Autodesk Inventor part; units mm, degrees
ref_plane "YZ Plane" through (0, 0, 0) normal (1, 0, 0) x (0, 1, 0)
ref_plane "XZ Plane" through (0, 0, 0) normal (0, 1, 0) x (-1, 0, 0)
ref_plane "XY Plane" through (0, 0, 0) normal (0, 0, 1) x (1, 0, 0)
sketch "Skizze1" plane through (0, 0, 0) normal (0, 0, 1) x (1, 0, 0)
  line L0 (-914, 455) -> (914, 455)
  line L1 (914, 455) -> (914, -455)
  line L2 (914, -455) -> (-914, -455)
  line L3 (-914, -455) -> (-914, 455)
  line L4 (-914, 455) -> (914, -455) construction
  line L5 (914, 455) -> (-914, -455) construction
  line L6 (-901.5, -442.5) -> (901.5, -442.5)
  line L7 (901.5, -442.5) -> (901.5, 442.5)
  line L8 (901.5, 442.5) -> (-901.5, 442.5)
  line L9 (-901.5, 442.5) -> (-901.5, -442.5)
  line L10 (-901.5, -442.5) -> (901.5, 442.5) construction
  line L11 (901.5, -442.5) -> (-901.5, 442.5) construction
  point P0 (0, 0)
  dimension "d0" = 1828
  dimension "d1" = 910
  dimension "d2" = 1803
  dimension "d3" = 885
extrude "Extrusion1" add sketch "Skizze1" along normal blind 139
sketch "Skizze2" plane through (0, 0, 139) normal (0, 0, 1) x (1, 0, 0)
  line L0 (-901.5, 442.5) -> (901.5, 442.5)
  line L1 (-901.5, -442.5) -> (-901.5, 442.5)
  line L2 (901.5, -442.5) -> (-901.5, -442.5)
  line L3 (901.5, 442.5) -> (901.5, -442.5)
  point P0 (0, 0)
sketch "Skizze3" plane through (914, -455, 0) normal (1, 0, 0) x (0, 0, -1)
  line L0 (0, 910) -> (0, 0) construction
  line L1 (0, 910) -> (-139, 910) construction
  line L2 (-139, 0) -> (-139, 910) construction
  line L3 (0, 0) -> (-139, 0) construction
  line L4 (-120.6636, 910) -> (-120.6636, 570) construction
  line L5 (-94.9295, 910) -> (-94.9295, 365) construction
  line L6 (-139, 511.8346) -> (-124, 511.8346) construction
  line L7 (-139, 570) -> (-124, 570)
  line L8 (-124, 570) -> (-124, 365)
  line L9 (-124, 365) -> (-139, 365)
  line L10 (-139, 365) -> (-139, 570)
  point P0 (0, 455)
  dimension "d8" = 340
  dimension "d9" = 545
  dimension "d10" = 15
extrude "Extrusion3" cut sketch "Skizze3" against normal through all
properties part number "Frame" material "Holz (Birke)"
Design review of the part built by this model. Coordinates are the model's own, in mm. A direction names the side the tool comes from. Give positions to 0.01 mm unless a question says otherwise; leave off trailing zeros. Order: outer loops, then holes, each group sorted by start corner. A loop starts at its lowest first (then second) coordinate and runs counter-clockwise, first axis right, second up. Notation, with made-up numbers: (5.25, 27) -> (37.25, 27) arc R19 ccw to (37.25, 62) -> close; hole circle Ø8 at (11, 38). An arc over 180 degrees is marked (long way). Write item = value, one per line. Start each with the question number.
(1) We need section C-C on z = 42.5. Write out the cut boundary in (x, y).
(2) For faces 4 (the face through (13, 442.5, 69)), 5 (the face through (-13, 455, 69)), list the 3-axis set-ups (+Z, -Z, +X, -X, +Y, -Y) from which the entire face can be reached by the end or side of a thin tool; tool diameter is ignored.
(3) For pin 1 (4 mm diameter, centred on x = 910.5, y = 13, fed in from +Z), flat-tipped, find the tip position at first contact; note if it passes through.
(4) We need section B-B on y = -383.5. Write out the cut boundary in (x, z), plus the area to 4 significant figures.
(5) To check wall thickness, follow line 1 along X through (y, z) = (-0.5, 39); line 2 along Y through (x, z) = (-222, 61.5). State the ranges of each line that lie inside material, in increasing order.
(6) Mouldability with a two-part tool opening along X and no side actions: class faces 1 (the face through (-4, 449, 139)), 2 (the face through (-914, -6, 69)), 3 (the face through (-13, -442.5, 69)) as +X half, -X half, draft (parallel to the pull), parting line (faces both ways), or undercut.
(7) We need section A-A on x = 398.5. Write out the cut boundary in (y, z).
Numbers:
q1.outline = (-914, -455) -> (914, -455) -> (914, 455) -> (-914, 455) -> close; hole (-901.5, -442.5) -> (901.5, -442.5) -> (901.5, 442.5) -> (-901.5, 442.5) -> close
q2.face_4 = +Z, -Z
q2.face_5 = +Z, -Z, +X, -X, +Y
q3.pin_1 = 124
q4.outline = (-914, 0) -> (-901.5, 0) -> (-901.5, 139) -> (-914, 139) -> close; (901.5, 0) -> (914, 0) -> (914, 139) -> (901.5, 139) -> close
q4.area = 3,475 mm^2
q5.line_1 = -914 to -901.5, 901.5 to 914
q5.line_2 = -455 to -442.5, 442.5 to 455
q6.face_1 = draft
q6.face_2 = -X half
q6.face_3 = undercut
q7.outline = (-455, 0) -> (-442.5, 0) -> (-442.5, 139) -> (-455, 139) -> close; (442.5, 0) -> (455, 0) -> (455, 139) -> (442.5, 139) -> close
